from build123d import *
from build123d.topology import SkipClean

# Parameters (mm, degrees)
EXTRUDE_1_DEPTH          = 2.5
REVOLVE_1_ANGLE          = 70
EXTRUDE_2_DEPTH          = 20
EXTRUDE_2_DEPTH_BACK     = 20
SKETCH_4_R               = 2.5
SKETCH_4_R_2             = 1
CUT_EXTRUDE_1_DEPTH      = 18.25
CUT_EXTRUDE_1_DEPTH_BACK = 18.25
SKETCH_5_R               = 1
CUT_EXTRUDE_START        = -100
SKETCH_6_R               = 1
CUT_EXTRUDE_2_DEPTH      = 100
EXTRUDE_START            = -5
SKETCH_8_R               = 1
EXTRUDE_3_DEPTH          = 5
SKETCH_9_R               = 1.004563183
CUT_EXTRUDE_3_DEPTH      = 10
EXTRUDE_START_2          = 1
SKETCH_10_R              = 2.5
SKETCH_10_R_2            = 1
EXTRUDE_4_DEPTH          = 1
SKETCH_11_R              = 2.5
SKETCH_11_R_2            = 1
EXTRUDE_5_DEPTH          = 1
SKETCH_13_W              = 11.686063101
SKETCH_13_H              = 0.769389088
CUT_EXTRUDE_4_DEPTH      = 10
CUT_EXTRUDE_5_DEPTH      = 10
SKETCH_15_R              = 4.4
CUT_EXTRUDE_7_DEPTH      = 1.75


with BuildPart() as part:
    # Sketch 1 → Extrude 1 (new body)
    with BuildSketch(Plane.XY):
        with BuildLine():
            Line((-20, 0), (-16.5, 0))
            ThreePointArc((-16.5, 0), (0, -16.5), (16.5, 0))
            Line((16.5, 0), (20, 0))
            ThreePointArc((20, 0), (0, -20), (-20, 0))
        make_face()
    extrude(amount=EXTRUDE_1_DEPTH)

    # Sketch 2 → Revolve 1 (revolve)
    with BuildSketch(Plane(origin=(0, 0, 0), x_dir=(-1, 0, 0), z_dir=(0, 0, -1))):
        with BuildLine():
            Line((-18.25, 0), (-16.5, 0))
            ThreePointArc((-16.5, 0), (0, -16.5), (16.5, 0))
            Line((16.5, 0), (18.25, 0))
            ThreePointArc((18.25, 0), (0, -18.25), (-18.25, 0))
        make_face()
    revolve(axis=Axis((16.5, 0, 0), (1, 0, 0)), revolution_arc=REVOLVE_1_ANGLE)

    # Sketch 4 → Extrude 2 (add, two sides: drawn at the far end of the back side and taken through both)
    with BuildSketch(Plane(origin=(0, 0, 0), x_dir=(0, 0, -1), z_dir=(1, 0, 0)).offset(-EXTRUDE_2_DEPTH_BACK)):
        with Locations(Location((0, 0, 0), (0, 0, 340))):
            Circle(SKETCH_4_R)
        with Locations(Location((0, 0, 0), (0, 0, 340))):
            Circle(SKETCH_4_R_2, mode=Mode.SUBTRACT)
    extrude(amount=EXTRUDE_2_DEPTH + EXTRUDE_2_DEPTH_BACK)

    # Sketch 5 → Cut-Extrude 1 (cut, two sides: drawn at the far end of the back side and taken through both)
    with SkipClean():  # the faces are left unmerged after this step: merging them gives an invalid solid
        with BuildSketch(Plane(origin=(0, 0, 0), x_dir=(0, 0, -1), z_dir=(1, 0, 0)).offset(-CUT_EXTRUDE_1_DEPTH_BACK)):
            with BuildLine():
                Line((0, -2.5), (-2.5, -2.5))
                Line((-2.5, -2.5), (-2.5, 0))
                ThreePointArc((-2.5, 0), (1.767766953, 1.767766953), (0, -2.5))
            make_face()
            Circle(SKETCH_5_R, mode=Mode.SUBTRACT)
        extrude(amount=CUT_EXTRUDE_1_DEPTH + CUT_EXTRUDE_1_DEPTH_BACK, mode=Mode.SUBTRACT)

    # Sketch 6 → Cut-Extrude 2 (cut)
    with SkipClean():  # the faces are left unmerged after this step: merging them gives an invalid solid
        with BuildSketch(Plane(origin=(20, 0, 0), x_dir=(0, 0, -1), z_dir=(1, 0, 0)).offset(CUT_EXTRUDE_START)):
            Circle(SKETCH_6_R)
        extrude(amount=CUT_EXTRUDE_2_DEPTH, mode=Mode.SUBTRACT)

    # Sketch 8 → Extrude 3 (add)
    with BuildSketch(Plane(origin=(20, 0, 0), x_dir=(0, 0, -1), z_dir=(1, 0, 0)).offset(EXTRUDE_START)):
        with BuildLine():
            ThreePointArc((2.494892647, -0.15972063), (0.003121638, -2.499998051), (-2.494485996, -0.165950649))
            Line((-2.494485996, -0.165950649), (-2.494485996, -8.665950649))
            Line((-2.494485996, -8.665950649), (2.505514004, -8.665950649))
            Line((2.505514004, -8.665950649), (2.494892647, -0.15972063))
        make_face()
        with Locations((0, -7)):
            Circle(SKETCH_8_R, mode=Mode.SUBTRACT)
    extrude(amount=EXTRUDE_3_DEPTH)

    # Sketch 9 → Cut-Extrude 3 (cut)
    with BuildSketch(Plane(origin=(20, 0, 0), x_dir=(0, 0, -1), z_dir=(1, 0, 0))):
        with Locations((0, -7)):
            Circle(SKETCH_9_R)
    extrude(amount=-CUT_EXTRUDE_3_DEPTH, mode=Mode.SUBTRACT)

    # Sketch 10 → Extrude 4 (add)
    with SkipClean():  # the faces are left unmerged after this step: merging them gives an invalid solid
        with BuildSketch(Plane.ZY.offset(20).offset(EXTRUDE_START_2)):
            Circle(SKETCH_10_R)
            with Locations(Location((0, 0, 0), (0, 0, 180))):
                Circle(SKETCH_10_R_2, mode=Mode.SUBTRACT)
        extrude(amount=-EXTRUDE_4_DEPTH)

    # Sketch 11 → Extrude 5 (add)
    with SkipClean():  # the faces are left unmerged after this step: merging them gives an invalid solid
        with BuildSketch(Plane(origin=(20, 0, 0), x_dir=(0, 0, -1), z_dir=(1, 0, 0))):
            Circle(SKETCH_11_R)
            Circle(SKETCH_11_R_2, mode=Mode.SUBTRACT)
        extrude(amount=EXTRUDE_5_DEPTH)

    # Sketch 12 → Cut-Revolve 1 (revolve, cut)
    with SkipClean():  # the faces are left unmerged after this step: merging them gives an invalid solid
        with BuildSketch(Plane.XY):
            with BuildLine():
                Line((-16.5, 0), (16.5, 0))
                ThreePointArc((16.5, 0), (0, -16.5), (-16.5, 0))
            make_face()
        revolve(axis=Axis((-16.5, 0, 0), (1, 0, 0)), mode=Mode.SUBTRACT)

    # Sketch 13 → Cut-Extrude 4 (cut)
    with SkipClean():  # the faces are left unmerged after this step: merging them gives an invalid solid
        with BuildSketch(Plane(origin=(0, 0.003115009, -2.494689321), x_dir=(-1, 0, 0), z_dir=(0, 0.00124865529263255, -0.9999992204296763))):
            with Locations((-12.40696845, -0.547530311)):
                Rectangle(SKETCH_13_W, SKETCH_13_H)
        extrude(amount=-CUT_EXTRUDE_4_DEPTH, mode=Mode.SUBTRACT)

    # Sketch 14 → Cut-Extrude 5 (cut)
    with SkipClean():  # the faces are left unmerged after this step: merging them gives an invalid solid
        with BuildSketch(Plane.ZY.offset(-18.25)):
            Polygon((-0.003121638, 1.949e-06), (2.5, 1.949e-06), (2.5, -2.5), (-0.003121638, -2.499998051), align=None)
        extrude(amount=CUT_EXTRUDE_5_DEPTH, mode=Mode.SUBTRACT)

    # Sketch 15 → Cut-Extrude 7 (cut)
    with SkipClean():  # the faces are left unmerged after this step: merging them gives an invalid solid
        with BuildSketch(Plane(origin=(20, 0, 0), x_dir=(0, 0, -1), z_dir=(1, 0, 0))):
            with Locations((0, -7)):
                Circle(SKETCH_15_R)
        extrude(amount=-CUT_EXTRUDE_7_DEPTH, mode=Mode.SUBTRACT)


solid = part.part
Can you work these out from the model? Positions are in its coordinate system, mm. A direction names the side the tool comes from. Round coordinates to 2 decimals unless told otherwise and drop trailing zeros. Loops run counter-clockwise (first coordinate to the right, second up) from the corner with the lowest first, then second, coordinate; pieces in that order, holes last. Notation, with made-up numbers: (-18, -10.5) - (2, -10.5) arc R19 cw to (2, 8.5) - close; hole circle Ø5 at (81.25, 82). An arc over 180 degrees is marked (long way). Answer in a Markdown table with one row per item. Add a question column.
Q1. We'd pull the mould along X, two halves only. Please class faces 4 (the cylindrical face through (-17.2, -2, -1.5)), 5 (the cylindrical face through (-3.81, -19.634, 1.232)), 6 (the cylindrical face through (16.37, -7.98, 0.22)): pulls with the +X half, pulls with the -X half, needs draft (parallel to the pull), parting line crosses it, or undercut.
Q2. I want a section at C-C on y = -12.5. List the corners of the cut face in (x, z) for me.
Q3. I need wall thicknesses on L1, parallel to Z at x = -19.35, y = 0; L2, parallel to X at y = -6.5, z = -4. Which ranges of each line are inside material? Lowest first, please.
Q4. I want a section at B-B on x = -3.5. List the corners of the cut face in (y, z) for me.
Q5. Which directions (+Z, -Z, +X, -X, +Y, -Y) give clear straight access to the entire face, cutting with the end or side of a thin tool? Please do faces 1 (the flat face through (-17, -2.5, 1)), 2 (the flat face through (-2.2, -18.3, 0)), 3 (the flat face through (-18.25, -1, 1)).
Q6. For pin 1 Ø10 at (x, y) = (-15.5, -5.5) entering from +Z; pin 2 Ø1.5 at (x, z) = (-16, -2) entering from -Y; pin 3 Ø1.5 at (y, z) = (-5.5, 1) entering from +X; pin 4 Ø8 at (y, z) = (-13.5, -14.5) entering from +X, each with a flat end and sliding along its axis, tell me the tip position at first contact or that it passes through.
A:
| question | item | result |
|---|---|---|
| 1 | face 4 | undercut |
| 1 | face 5 | parting line crosses it |
| 1 | face 6 | needs draft |
| 2 | outline | (-15.61, 0) - (-13.3, 0) arc R13.3 ccw to (13.3, 0) - (15.61, 0) - (15.61, 2.5) - (10.77, 2.5) - (10.77, 0) arc R10.77 cw to (-10.77, 0) - (-10.77, 2.5) - (-15.61, 2.5) - close |
| 3 | L1 | -2.5 to -1, 1 to 2.5 |
| 3 | L2 | -16.58 to -14.63, 14.63 to 16.58 |
| 4 | outline | (-19.69, 0) - (-17.91, 0) arc R17.91 ccw to (-6.13, -16.83) - (-5.51, -15.15) arc R16.12 cw to (-16.12, 0) - (-16.12, 2.5) - (-19.69, 2.5) - close |
| 5 | face 1 | +Z, +Y |
| 5 | face 2 | -Z, -Y |
| 5 | face 3 | +Z, -Z, +Y |
| 6 | pin 1 | z = 2.5 |
| 6 | pin 2 | y = -9.83 |
| 6 | pin 3 | x = 18.25 |
| 6 | pin 4 | x = 9.11 |
